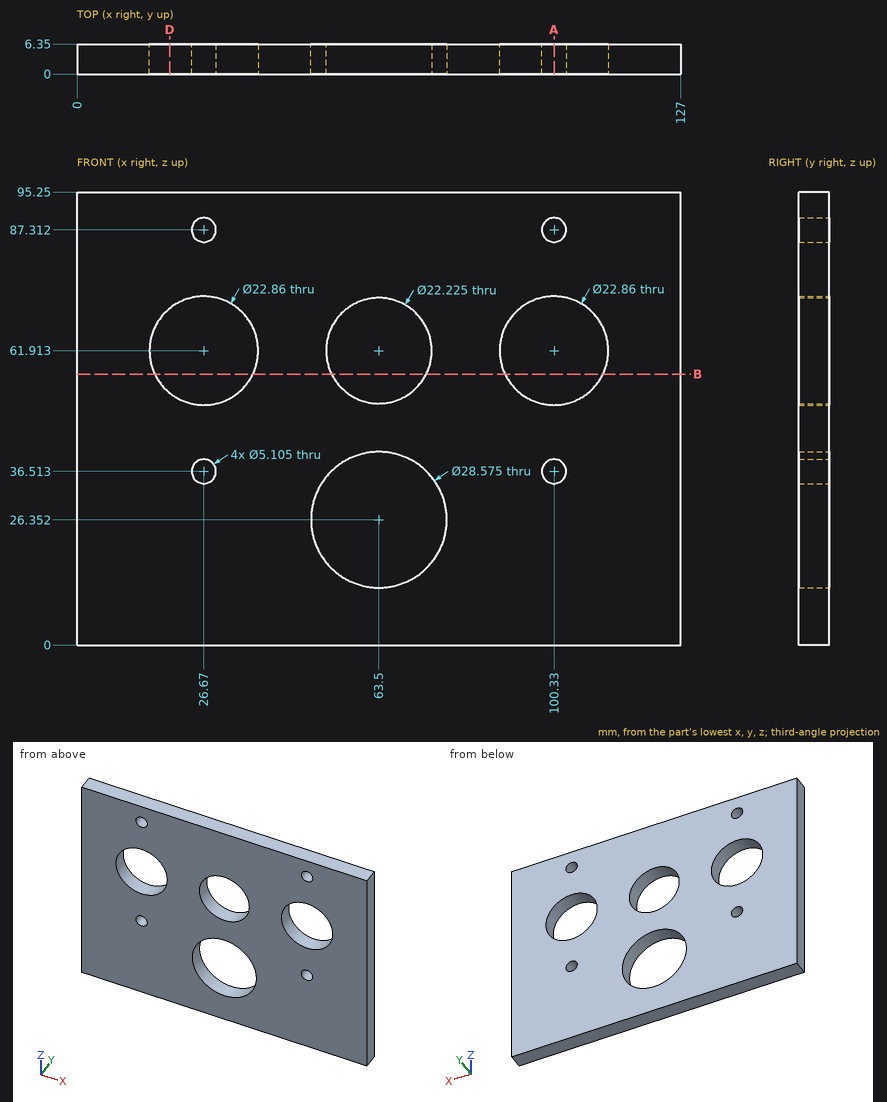
Geometry: see drawing. Coordinates: mm, zero at the bounding-box minimum. Round coordinates to 2 decimals unless told otherwise and drop trailing zeros. Write each loop counter-clockwise with the first axis right and the second up, starting at its lowest first coordinate (ties: lowest second). Pieces come first, ordered by that corner, then holes.
Item 1: Section query B-B (z = 57). Return loops of the section in (x, y), plus the area to 3 significant figures.
Item 2: Material intervals for L1, parallel to X at y = 1.25, z = 31; L2, parallel to X at y = 4, z = 64.5; L3, parallel to X at y = 4.25, z = 29, sorted ascending.
Item 3: Section query D-D (x = 19.5). Return loops of the section in (y, z).
Item 4: Section query A-A (x = 100.33). Give the number of separate pieces and of enclosed holes in the cut face, plus the area to 3 significant figures.
Completed:
1. outline: (0, 0) - (16.35, 0) - (16.35, 6.35) - (0, 6.35) - close; (36.99, 0) - (53.53, 0) - (53.53, 6.35) - (36.99, 6.35) - close; (73.47, 0) - (90.01, 0) - (90.01, 6.35) - (73.47, 6.35) - close; (110.65, 0) - (127, 0) - (127, 6.35) - (110.65, 6.35) - close
1. area: 418 mm2
2. L1: x = 0 to 49.99, 77.01 to 127
2. L2: x = 0 to 15.54, 37.8 to 52.69, 74.31 to 89.2, 111.46 to 127
2. L3: x = 0 to 49.46, 77.54 to 127
3. outline: (0, 0) - (6.35, 0) - (6.35, 53.01) - (0, 53.01) - close; (0, 70.81) - (6.35, 70.81) - (6.35, 95.25) - (0, 95.25) - close
4. separate pieces: 4
4. enclosed holes: 0
4. area: 395 mm2
